Autodesk Inventor part; units mm, degrees
ref_plane "YZ Plane" through (0, 0, 0) normal (1, 0, 0) x (0, 1, 0)
ref_plane "XZ Plane" through (0, 0, 0) normal (0, 1, 0) x (-1, 0, 0)
ref_plane "XY Plane" through (0, 0, 0) normal (0, 0, 1) x (1, 0, 0)
sketch "Sketch1" plane through (0, 0, 0) normal (0, 1, 0) x (-1, 0, 0)
  line L0 (0, 0) -> (0, -412)
  line L1 (0, -412) -> (6.35, -412)
  line L2 (6.35, -412) -> (6.35, 0)
  line L3 (6.35, 0) -> (0, 0)
  dimension "d0" = 412
  dimension "d1" = 6.35
extrude "Extrusion1" add sketch "Sketch1" along normal blind 6.35
sketch "Sketch2" plane through (0, 6.35, 0) normal (0, 1, 0) x (1, 0, 0)
  point P0 (0, 0)
sketch "Sketch3" plane through (-6.35, 0, -412) normal (-1, 0, 0) x (0, 0, 1)
  line L0 (412, 6.35) -> (0, 6.35)
  point P0 (412, 0)
sketch "Sketch4" plane through (-6.35, 0, -412) normal (-1, 0, 0) x (0, 0, 1)
  line L0 (412, 6.35) -> (403.5733, 0)
  line L1 (412, 0) -> (0, 0)
  line L2 (412, 6.35) -> (422.5514, 6.35) construction
  line L3 (403.5733, 0) -> (412, 0)
  line L4 (412, 0) -> (412, 6.35)
  dimension "d6" = 143
extrude "Extrusion2" cut sketch "Sketch4" against normal blind 10
sketch "Sketch5" plane through (-6.35, 0, -412) normal (-1, 0, 0) x (0, 0, 1)
  line L0 (0, 6.35) -> (8.4267, 0)
  line L1 (0, 6.35) -> (10.5514, 6.35) construction
  line L2 (8.4267, 0) -> (0, 0)
  line L3 (0, 6.35) -> (412, 6.35)
  line L4 (0, 0) -> (0, 6.35)
  point P0 (412, 0)
  dimension "d9" = 37
extrude "Extrusion3" cut sketch "Sketch5" against normal blind 10
sketch "Sketch6" plane through (-6.35, 0, -403.5733) normal (-1, 0, 0) x (0, 0, 1)
  line L0 (403.5733, 6.35) -> (-8.4267, 6.35)
  line L1 (403.5733, 6.35) -> (403.5733, 0)
  line L2 (403.5733, 6.35) -> (395.1465, 0)
  line L3 (403.5733, 0) -> (395.1465, 0)
  line L4 (395.1465, 0) -> (403.5733, 6.35)
extrude "Extrusion4" add sketch "Sketch6" against normal blind 6.35
sketch "Sketch7" plane through (-6.35, 6.35, -412) normal (-1, 0, 0) x (0, 0, 1)
  line L0 (8.4267, -6.35) -> (412, -6.35)
  line L1 (8.4267, -6.35) -> (0, -6.35)
  line L2 (0, 0) -> (412, 0)
  line L3 (0, -6.35) -> (0, 0)
  line L4 (0, 0) -> (8.4267, -6.35)
extrude "Extrusion5" add sketch "Sketch7" against normal blind 6.35
sketch "Sketch8" plane through (0, 6.35, 0) normal (0, 1, 0) x (1, 0, 0)
  line L0 (-6.35, 0) -> (0, 0)
  line L1 (0, 0) -> (-6.35, 8.4267)
  line L2 (0, 0) -> (10.5514, 0) construction
  line L3 (-6.35, 8.4267) -> (-6.35, 0)
  line L4 (-6.35, 0) -> (0, 0)
  dimension "d16" = 127
extrude "Extrusion6" cut sketch "Sketch8" against normal blind 10
sketch "Sketch9" plane through (0, 6.35, 0) normal (0, 1, 0) x (1, 0, 0)
  line L0 (0, 412) -> (-6.3367, 403.5909)
  line L1 (0, 412) -> (10.5293, 412) construction
  line L2 (-6.3367, 403.5909) -> (-6.3367, 412)
  line L3 (0, 0) -> (0, 412)
  line L4 (-6.3367, 412) -> (0, 412)
  dimension "d19" = 127
extrude "Extrusion7" cut sketch "Sketch9" against normal blind 10
properties part number "Main"
Input: part model. Units: mm. Frame: model coordinates. Coordinates: 2 decimals unless noted, no trailing zeros. Loops run counter-clockwise (first coordinate to the right, second up) from the corner with the lowest first, then second, coordinate; pieces in that order, holes last. Notation, with made-up numbers: (-34, -37.5) -> (14, -37.5) arc R8 cw to (14, -33.5) -> close; hole circle Ø4 at (47, 29). An arc over 180 degrees is marked (long way). One line per item, written item: value.
(1) Ray query, line 1 along Z through (x, y) = (-5, 4.5); line 2 along Z through (x, y) = (-4.5, 5). Return the intervals inside material, ascending.
Answer below:
line 1: z = -405.36 to -6.64
line 2: z = -406.03 to -5.97
(2) Cut plane B-B (x = -3.5). Output: boundary loops of the cut face in (y, z).
Answer below:
outline: (0, -407.36) -> (6.35, -407.36) -> (6.35, -4.64) -> (0, -4.64) -> close
(3) Pin query (flat end, axial travel): pin 1 Ø1 at (x, y) = (-1, 3) entering from -Z; pin 2 Ø3 at (x, y) = (-0.5, 1.5) entering from +Z. Return the tip coordinate at first contact, or that it passes through.
Answer below:
pin 1: stops at z = -411.34
pin 2: stops at z = 0
